Autodesk Inventor part; units mm, degrees
ref_plane "YZ Plane" through (0, 0, 0) normal (1, 0, 0) x (0, 1, 0)
ref_plane "XZ Plane" through (0, 0, 0) normal (0, 1, 0) x (-1, 0, 0)
ref_plane "XY Plane" through (0, 0, 0) normal (0, 0, 1) x (1, 0, 0)
sketch "スケッチ1" plane through (0, 0, 0) normal (0, 0, 1) x (1, 0, 0)
  line L0 (0, 0) -> (38, 0)
  line L1 (38, 0) -> (38, 104)
  line L2 (38, 104) -> (0, 104)
  line L3 (0, 104) -> (0, 0)
  dimension "d0" = 38
  dimension "d1" = 104
extrude "押し出し1" add sketch "スケッチ1" along normal blind 2
sketch "スケッチ2" plane through (0, 0, 2) normal (0, 0, 1) x (1, 0, 0)
  line L0 (38, 104) -> (0, 104)
  line L1 (0, 0) -> (38, 0)
  line L2 (38, 0) -> (38, 104)
  line L3 (38, 104) -> (0, 104)
  line L4 (0, 104) -> (0, 0)
  line L5 (2.9, 0) -> (35.1, 0)
  line L6 (35.1, 0) -> (35.1, 104)
  line L7 (35.1, 104) -> (2.9, 104)
  line L8 (2.9, 104) -> (2.9, 0)
  point P0 (2.9, 0)
  dimension "d4" = 2.9
  dimension "d5" = 2.9
  dimension "d6" = 0
  dimension "d7" = 0
extrude "押し出し2" add sketch "スケッチ2" along normal blind 5 contours L2 L1 L6 L0 | L8 L1 L4 L0
sketch "スケッチ3" plane through (0, 0, 0) normal (0, 0, -1) x (-1, 0, 0)
  line L0 (-38, 104) -> (0, 104)
  line L1 (0, 0) -> (-38, 0)
  line L2 (-35.1, 0) -> (-35.1, 104)
  line L3 (-2.9, 104) -> (-2.9, 0)
  point P0 (-32.5, 99)
  point P1 (-5.5, 99)
  point P2 (-5.5, 5)
  point P3 (-32.5, 5)
  dimension "d10" = 5
  dimension "d11" = 5
  dimension "d12" = 5
  dimension "d13" = 5
  dimension "d14" = 27
  dimension "d15" = 2.6
  dimension "d16" = 27
  dimension "d17" = 2.6
hole "穴1" at (32.5, 99, 0) at (5.5, 99, 0) at (5.5, 5, 0) at (32.5, 5, 0) direction (0, 0, 1) diameter 3.2 end through all
sketch "スケッチ4" plane through (0, 0, 0) normal (0, 0, -1) x (-1, 0, 0)
  circle A0 centre (-32.5, 99) radius 1.6
  circle A1 centre (-5.5, 99) radius 1.6
  circle A2 centre (-32.5, 5) radius 1.6
  line L0 (0, 104) -> (0, 0)
  line L1 (0, 0) -> (-38, 0)
  circle A3 centre (-32.5, 99) radius 4
  circle A4 centre (-5.5, 99) radius 4
  circle A5 centre (-32.5, 5) radius 4
  circle A6 centre (-5.5, 5) radius 1.6
  circle A7 centre (-5.5, 5) radius 4
  point P0 (-5.5, 15)
  dimension "d25" = 5.5
  dimension "d26" = 15
  dimension "d27" = 8
  dimension "d28" = 8
  dimension "d29" = 8
  dimension "d30" = 8
extrude "押し出し3" cut sketch "スケッチ4" against normal blind 1
sketch "スケッチ5" plane through (0, 0, 2) normal (0, 0, 1) x (1, 0, 0)
  line L0 (2.9, 104) -> (2.9, 0)
  line L1 (35.1, 0) -> (35.1, 104)
  line L2 (2.9, 8.3) -> (35.1, 8.3)
  line L3 (35.1, 8.3) -> (35.1, 11.3)
  line L4 (35.1, 11.3) -> (2.9, 11.3)
  line L5 (2.9, 11.3) -> (2.9, 8.3)
  line L6 (2.9, 95.7) -> (35.1, 95.7)
  line L7 (35.1, 95.7) -> (35.1, 92.7)
  line L8 (35.1, 92.7) -> (2.9, 92.7)
  line L9 (2.9, 92.7) -> (2.9, 95.7)
  circle A0 centre (32.5, 5) radius 1.6
  circle A1 centre (5.5, 5) radius 1.6
  circle A2 centre (5.5, 99) radius 1.6
  circle A3 centre (32.5, 99) radius 1.6
  line L10 (2.9, 104) -> (2.9, 0)
  line L11 (2.9, 0) -> (35.1, 0)
  line L12 (35.1, 0) -> (35.1, 104)
  line L13 (35.1, 104) -> (2.9, 104)
  point P0 (0, 0)
  point P1 (2.9, 11.3)
  point P2 (2.9, 92.7)
  point P3 (2.9, 95.7)
  dimension "d33" = 3
  dimension "d34" = 3
  dimension "d35" = 3.3
  dimension "d36" = 3.3
extrude "押し出し4" add sketch "スケッチ5" along normal blind 5 contours L6 L1 L8 L0 | L4 L1 L2 L0
properties part number "robot-arm-frame"
Build history of the part. All positions in model axes, mm. A direction names the side the tool comes from. Round coordinates to 2 decimals unless told otherwise and drop trailing zeros. Write each loop counter-clockwise with the first axis right and the second up, starting at its lowest first coordinate (ties: lowest second). Pieces come first, ordered by that corner, then holes. Notation, with made-up numbers: (5, 24) -> (19, 24) arc R21 ccw to (19, 53) -> close; hole circle Ø1 at (3.5, 6.25). An arc over 180 degrees is marked (long way). Use one line per item in the form item = value.
Q1. Tool access for faces 1 (the flat face through (35.1, 51, 4)), 2 (the flat face through (19, 8.3, 4)), 3 (the flat face through (2.9, 100, 4)): list every direction of +Z, -Z, +X, -X, +Y, -Y with a clear straight run to the whole face (end or side of a thin tool).
Conclusion:
face_1 = +Z
face_2 = +Z, -Y
face_3 = +Z, +Y
Q2. Band-saw the part on B-B, the plane y = 99. Write the cut outline in (x, z).
Conclusion:
outline = (0, 0) -> (1.5, 0) -> (1.5, 1) -> (3.9, 1) -> (3.9, 2) -> (2.9, 2) -> (2.9, 7) -> (0, 7) -> close; (7.1, 1) -> (9.5, 1) -> (9.5, 0) -> (28.5, 0) -> (28.5, 1) -> (30.9, 1) -> (30.9, 2) -> (7.1, 2) -> close; (34.1, 1) -> (36.5, 1) -> (36.5, 0) -> (38, 0) -> (38, 7) -> (35.1, 7) -> (35.1, 2) -> (34.1, 2) -> close
Q3. Two-plate mould, pull along Y, no slides. Class faces 4 (the flat face through (19, 104, 1)), 5 (the flat face through (36, 52, 7)), 6 (the cylindrical face through (33.367, 95.095, 0.493)): released by +Y, released by -Y, zero draft, split by the parting line, or undercut.
Conclusion:
face_4 = released by +Y
face_5 = zero draft
face_6 = undercut
Q4. Drop flat-ended pins along their axis: P1, Ø2.5, axis at x = 32, y = 98, coming from the -Z side; P2, Ø3, axis at x = 8.5, y = 72.5, coming from the +Z side; P3, Ø2.5, axis at x = 22.5, z = 5.5, coming from the +Y side. Give the stop position or say it passes through.
Conclusion:
P1 = 1
P2 = 2
P3 = 95.7
Q5. Band-saw the part on A-A, the plane x = 5.5. Write the cut outline in (y, z).
Conclusion:
outline = (0, 0) -> (1, 0) -> (1, 1) -> (3.4, 1) -> (3.4, 2) -> (0, 2) -> close; (6.6, 1) -> (9, 1) -> (9, 0) -> (95, 0) -> (95, 1) -> (97.4, 1) -> (97.4, 2) -> (95.7, 2) -> (95.7, 7) -> (92.7, 7) -> (92.7, 2) -> (11.3, 2) -> (11.3, 7) -> (8.3, 7) -> (8.3, 2) -> (6.6, 2) -> close; (100.6, 1) -> (103, 1) -> (103, 0) -> (104, 0) -> (104, 2) -> (100.6, 2) -> close
Q6. Band-saw the part on C-C, the plane z = 5.75. Write the cut outline in (x, y), then the cut area to 3 significant figures.
Conclusion:
outline = (0, 0) -> (2.9, 0) -> (2.9, 8.3) -> (35.1, 8.3) -> (35.1, 0) -> (38, 0) -> (38, 104) -> (35.1, 104) -> (35.1, 95.7) -> (2.9, 95.7) -> (2.9, 104) -> (0, 104) -> close; hole (2.9, 11.3) -> (35.1, 11.3) -> (35.1, 92.7) -> (2.9, 92.7) -> close
area = 796 mm²
Q7. Band-saw the part on D-D, the plane y = 65. Write the cut outline in (x, z).
Conclusion:
outline = (0, 0) -> (38, 0) -> (38, 7) -> (35.1, 7) -> (35.1, 2) -> (2.9, 2) -> (2.9, 7) -> (0, 7) -> close
Q8. Drill centre lines: L1, parallel to Y at x = 5.5, z = 1.8; L2, parallel to X at y = 99, z = 1.25; L3, parallel to Y at x = 5.5, z = 0.65. Where is each one in solid material? Low to high.
Conclusion:
L1 = 0 to 3.4, 6.6 to 97.4, 100.6 to 104
L2 = 0 to 3.9, 7.1 to 30.9, 34.1 to 38
L3 = 0 to 1, 9 to 95, 103 to 104
